Geometry check sheet. Reference: the model listing, model coordinates, mm. Face numbers are marked on the shaded views. Give positions to 0.01 mm unless a question says otherwise; leave off trailing zeros. Write each loop counter-clockwise with the first axis right and the second up, starting at its lowest first coordinate (ties: lowest second). Pieces come first, ordered by that corner, then holes. Notation, with made-up numbers: M 35,6.5 L 70,6.5 A13 cw 70,15.5 Z; hole C 80.5,0.5 d8. An arc over 180 degrees is marked long. Use one line per item in the form item = value. Start each with the question number.
Autodesk Fusion 360 part; units mm, degrees
sketch "sketch_base_outline" plane through (0, 0, 0) normal (0, 0, 1) x (1, 0, 0)
  line L0 (0, 0) -> (100, 0)
  line L1 (100, 0) -> (100, 60)
  line L2 (100, 60) -> (0, 60)
  line L3 (0, 60) -> (0, 0)
extrude "Extrude1" add sketch "sketch_base_outline" along normal blind 10
sketch "sketch_inner_pocket" plane through (0, 0, 10) normal (0, 0, 1) x (1, 0, 0)
  line L0 (0, 60) -> (0, 0)
  line L1 (0, 0) -> (100, 0)
  line L2 (100, 0) -> (100, 60)
  line L3 (100, 60) -> (0, 60)
  line L4 (25, 15) -> (75, 15)
  line L5 (75, 15) -> (75, 45)
  line L6 (75, 45) -> (25, 45)
  line L7 (25, 45) -> (25, 15)
sketch "sketch_bore_hole" plane through (0, 0, 10) normal (0, 0, 1) x (1, 0, 0)
  line L0 (0, 60) -> (0, 0)
  line L1 (0, 0) -> (100, 0)
  line L2 (100, 0) -> (100, 60)
  line L3 (100, 60) -> (0, 60)
  circle A0 centre (82, 18) radius 6
extrude "bore_hole" cut sketch "sketch_bore_hole" against normal blind 10 contours A0
equation "d3 = -( 10 mm )"
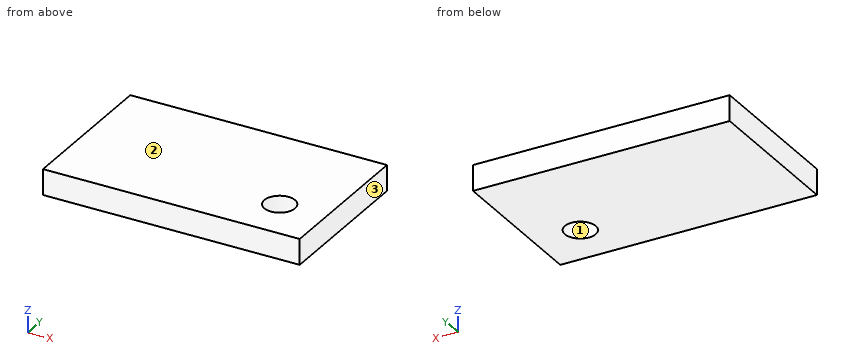
(1) Draft check along X on the marked faces 1, 2 and 3. Enter one of: released by +X, released by -X, zero draft, split by the parting line, or undercut.
(2) Sectioned sample at B-B, the plane x = 82. Record the boundary of the cut face in (y, z), plus the area to 3 significant figures.
(3) Depth check by flat-ended pin: pin 1 (9.5 mm diameter, centred on x = 82, y = 18, fed in from -Z). Enter the tip coordinate at first touch or a pass-through.
(4) Sectioned sample at A-A, the plane y = 18. Record the boundary of the cut face in (x, z), plus the area to 3 significant figures.
(5) Thickness scan on probe 1 along Y at (x, z) = (82, 6.75); probe 2 along Y at (x, z) = (78, 2.5). Record the ranges inside material, lowest first. Write a range as [from, to].
(6) Sectioned sample at C-C, the plane z = 7.5. Record the boundary of the cut face in (x, y), plus the area to 3 significant figures.
Numbers:
q1.face_1 = undercut
q1.face_2 = zero draft
q1.face_3 = released by +X
q2.outline = M 0,0 L 12,0 L 12,10 L 0,10 Z; M 24,0 L 60,0 L 60,10 L 24,10 Z
q2.area = 480 mm2
q3.pin_1 = through
q4.outline = M 0,0 L 76,0 L 76,10 L 0,10 Z; M 88,0 L 100,0 L 100,10 L 88,10 Z
q4.area = 880 mm2
q5.probe_1 = [0, 12], [24, 60]
q5.probe_2 = [0, 13.53], [22.47, 60]
q6.outline = M 0,0 L 100,0 L 100,60 L 0,60 Z; hole C 82,18 d12
q6.area = 5,890 mm2
